Input: dimensioned drawing with shaded views. Units: mm. Origin: part minimum x, y, z. Round coordinates to 2 decimals unless told otherwise and drop trailing zeros. Loops run counter-clockwise (first coordinate to the right, second up) from the corner with the lowest first, then second, coordinate; pieces in that order, holes last. Notation, with made-up numbers: M 52.25,48.5 L 80.25,48.5 A12 cw 80.25,63.5 Z; hole C -25,34 d3. An arc over 180 degrees is marked long. Put each result on its own line as item: value. Start each with the question number.
1) Pin query (flat end, axial travel): pin 1 (2.5 mm diameter, centred on x = 25.5, y = 40.9, fed in from +Z). Return the tip coordinate at first contact, or that it passes through.
2) Section A-A on z = 4.5. Output: boundary loops of the cut face in (x, y).
3) Line query: probe 1 along Y at (x, z) = (2.5, 3.4); probe 2 along X at (y, z) = (3, 1.25). Output: solid intervals per line, ascending.
4) Section C-C on y = 2.5. Output: boundary loops of the cut face in (x, z).
5) Section B-B on x = 2.5. Output: boundary loops of the cut face in (y, z), plus the area to 3 significant figures.
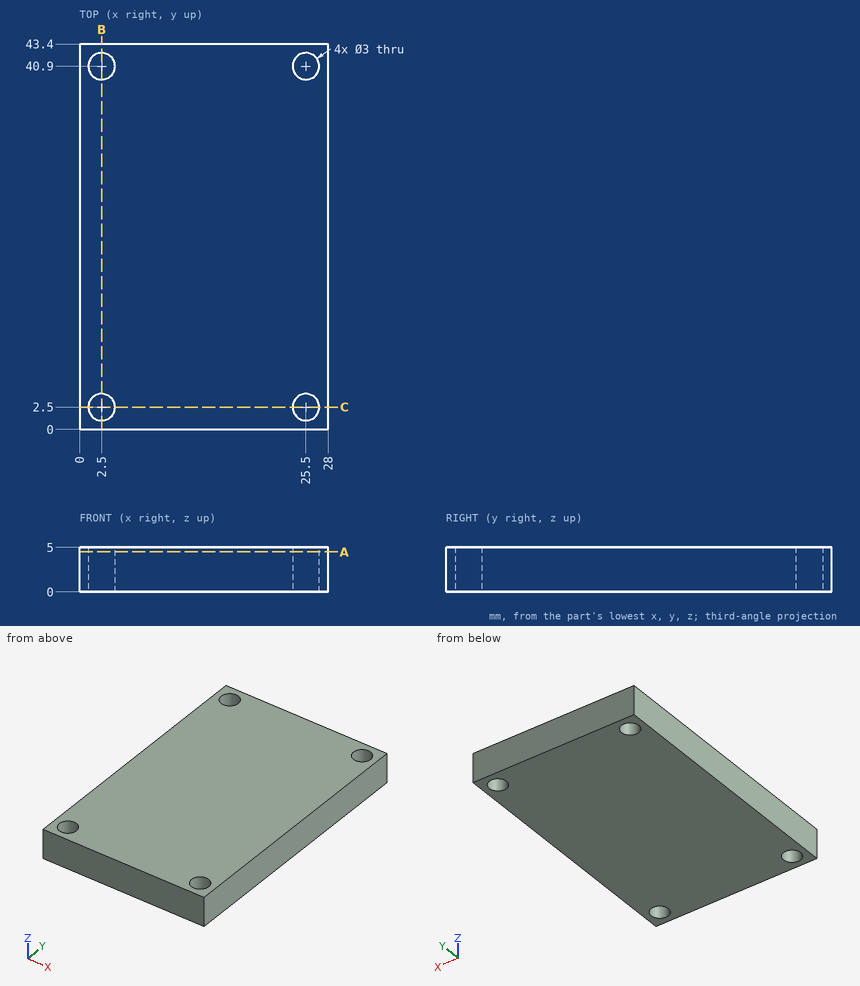
Geometry results:
1. pin 1: passes through
2. outline: M 0,0 L 28,0 L 28,43.4 L 0,43.4 Z; hole C 2.5,2.5 d3; hole C 2.5,40.9 d3; hole C 25.5,2.5 d3; hole C 25.5,40.9 d3
3. probe 1: y = 0 to 1, 4 to 39.4, 42.4 to 43.4
3. probe 2: x = 0 to 1.09, 3.91 to 24.09, 26.91 to 28
4. outline: M 0,0 L 1,0 L 1,5 L 0,5 Z; M 4,0 L 24,0 L 24,5 L 4,5 Z; M 27,0 L 28,0 L 28,5 L 27,5 Z
5. outline: M 0,0 L 1,0 L 1,5 L 0,5 Z; M 4,0 L 39.4,0 L 39.4,5 L 4,5 Z; M 42.4,0 L 43.4,0 L 43.4,5 L 42.4,5 Z
5. area: 187 mm²
